Check sheet for the modelled part. Datum: model origin and axes. Units: mm. Face numbers are marked on the shaded views. A direction names the side the tool comes from. Coordinates: 2 decimals unless noted, no trailing zeros. Loops run counter-clockwise (first coordinate to the right, second up) from the corner with the lowest first, then second, coordinate; pieces in that order, holes last. Notation, with made-up numbers: M -25,-3 L 5,-3 A11 ccw 5,10 Z; hole C 50,27 d10. An arc over 180 degrees is marked long. Use CSV: the item, a comma, the result in double quotes. Start each with the question number.
(1) Section check D-D on x = 48. Record the cut outline in (y, z).
(2) Section check A-A on z = -6.75. Record the cut outline in (x, y).
(3) Scan lines: line 1 (Y direction, x = 50, z = -3.5); line 2 (X direction, y = 20, z = -7); line 3 (Y direction, x = 81, z = -5.5). Record each from-to range of solid material in increasing order.
(4) Go/stop test with flat-tipped pins: pin 1 Ø6 at (x, z) = (131, -9.5) entering from +Y; pin 2 Ø5 at (y, z) = (43, -5) entering from +X; pin 3 Ø4 at (x, z) = (89.5, -8) entering from +Y; pin 4 Ø5.5 at (x, y) = (0, 100) entering from +Z. Record where each tip stops, or that it passes through.
(5) Set-up check for the marked faces 1, 2 and 3: record each of +Z, -Z, +X, -X, +Y, -Y from which the full face is reachable in a straight line by a thin tool's end or side.
(6) Section check B-B on z = -17.25. Record the cut outline in (x, y), and give its area (3 significant figures).
(7) Draft check along Y on the marked faces 4, 5, 6 and 7. Enter one of: pulls with the +Y half, pulls with the -Y half, needs draft (parallel to the pull), parting line crosses it, or undercut.
(8) Section check C-C on y = 50.5. Record the cut outline in (x, z).
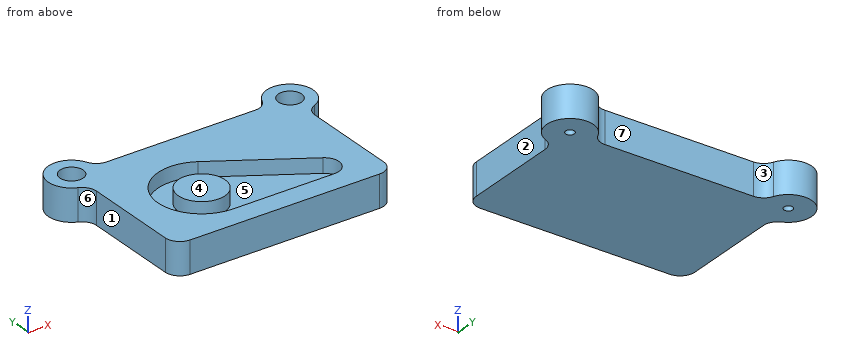
from build123d import *

# Parameters (mm, degrees)
SKETCH4_R          = 3
EXTRUDE1_DEPTH     = 22
SKETCH4_3_R        = 16
CUT_EXTRUDE1_DEPTH = 10
SKETCH4_4_R        = 8
CUT_EXTRUDE2_DEPTH = 10


with BuildPart() as part:
    # Sketch4 → Extrude1 (new body)
    with BuildSketch(Plane.XY):
        with BuildLine():
            Line((126, 100), (24, 100))
            ThreePointArc((24, 100), (18.452998038, 101.679497057), (14.769230769, 106.153846154))
            ThreePointArc((14.769230769, 106.153846154), (-11.313708499, 111.313708499), (-6.153846154, 85.230769231))
            ThreePointArc((-6.153846154, 85.230769231), (-1.679497057, 81.547001962), (0, 76))
            Line((0, 76), (0, 10))
            ThreePointArc((0, 10), (2.928932188, 2.928932188), (10, 0))
            Line((10, 0), (140, 0))
            ThreePointArc((140, 0), (147.071067812, 2.928932188), (150, 10))
            Line((150, 10), (150, 76))
            ThreePointArc((150, 76), (151.679497057, 81.547001962), (156.153846154, 85.230769231))
            ThreePointArc((156.153846154, 85.230769231), (161.313708499, 111.313708499), (135.230769231, 106.153846154))
            ThreePointArc((135.230769231, 106.153846154), (131.547001962, 101.679497057), (126, 100))
        make_face()
        with Locations((0, 100)):
            Circle(SKETCH4_R, mode=Mode.SUBTRACT)
        with Locations((150, 100)):
            Circle(SKETCH4_R, mode=Mode.SUBTRACT)
    extrude(amount=-EXTRUDE1_DEPTH)

    # Sketch4<3> → Cut-Extrude1 (cut)
    with BuildSketch(Plane.XY):
        with BuildLine():
            Line((65.849056604, 70.471698113), (125.283018868, 33.490566038))
            ThreePointArc((125.283018868, 33.490566038), (129.615239476, 22.252788721), (120, 15))
            Line((120, 15), (50, 15))
            ThreePointArc((50, 15), (21.154281571, 53.241633837), (65.849056604, 70.471698113))
        make_face()
        with Locations((50, 45)):
            Circle(SKETCH4_3_R, mode=Mode.SUBTRACT)
    extrude(amount=-CUT_EXTRUDE1_DEPTH, mode=Mode.SUBTRACT)

    # Sketch4<4> → Cut-Extrude2 (cut)
    with BuildSketch(Plane.XY):
        with Locations((0, 100)):
            Circle(SKETCH4_4_R)
        with Locations((150, 100)):
            Circle(SKETCH4_4_R)
    extrude(amount=-CUT_EXTRUDE2_DEPTH, mode=Mode.SUBTRACT)


solid = part.part
Outcome:
1,outline,"M 0,-22 L 100,-22 L 100,0 L 74.93,0 L 74.93,-10 L 60.87,-10 L 60.87,0 L 29.13,0 L 29.13,-10 L 15.07,-10 L 15.07,0 L 0,0 Z"
2,outline,"M -6.15,85.23 A10 cw 0,76 L 0,10 A10 ccw 10,0 L 140,0 A10 ccw 150,10 L 150,76 A10 cw 156.15,85.23 A16 ccw long 135.23,106.15 A10 cw 126,100 L 24,100 A10 cw 14.77,106.15 A16 ccw long Z; C 50,45 d32; hole C 0,100 d16; hole M 50,15 L 120,15 A10 ccw 125.28,33.49 L 65.85,70.47 A30 ccw long Z; hole C 150,100 d16"
3,line 1,"y = 0 to 15, 29 to 61, 75 to 100"
3,line 2,"x = 0 to 33.42, 128.66 to 150"
3,line 3,"y = 0 to 15, 61.04 to 100"
4,pin 1,"stops at y = 104"
4,pin 2,"stops at x = 150"
4,pin 3,"stops at y = 100"
4,pin 4,"passes through"
5,face 1,"+Z, -Z, -X, -Y"
5,face 2,"+Z, -Z, +X, -Y"
5,face 3,"+Z, -Z, +Y"
6,outline,"M -6.15,85.23 A10 cw 0,76 L 0,10 A10 ccw 10,0 L 140,0 A10 ccw 150,10 L 150,76 A10 cw 156.15,85.23 A16 ccw long 135.23,106.15 A10 cw 126,100 L 24,100 A10 cw 14.77,106.15 A16 ccw long Z; hole C 0,100 d6; hole C 150,100 d6"
6,area,"16,100 mm²"
7,face 4,"needs draft"
7,face 5,"undercut"
7,face 6,"pulls with the -Y half"
7,face 7,"pulls with the +Y half"
8,outline,"M 0,-22 L 150,-22 L 150,0 L 97.95,0 L 97.95,-10 L 65.02,-10 L 65.02,0 L 34.98,0 L 34.98,-10 L 20.51,-10 L 20.51,0 L 0,0 Z"
